Could you check a few things on this model? Use its own coordinates, in mm. Face numbers are marked on the shaded views. A direction names the side the tool comes from. Coordinates: 2 decimals unless noted, no trailing zeros. Order: outer loops, then holes, each group sorted by start corner. A loop starts at its lowest first (then second) coordinate and runs counter-clockwise, first axis right, second up. Notation, with made-up numbers: (-37.5, 64.25) - (-6.5, 64.25) arc R26 cw to (-6.5, 94.25) - close; hole circle Ø6 at (76.5, -26.5). An arc over 180 degrees is marked (long way). Answer as CSV lines item,"result". Start each with the question number.
1. For pin 1 (1.6 mm diameter, centred on x = 0, z = 0, fed in from +Y); pin 2 (2 mm diameter, centred on y = 6, z = -0.5, fed in from +X), each with a flat end and sliding along its axis, tell me the tip position at first contact or that it passes through.
2. Thinking about a two-plate mould opening in X: for the marked faces 3, 4 and 5, which applies, released by +X, released by -X, zero draft, split by the parting line, or undercut?
3. I want a section at A-A, the plane x = 0. List the corners of the cut face in (y, z) for me (3 decimals).
4. I want a section at B-B, the plane y = 1.5. List the corners of the cut face in (x, z) for me, and give its area (3 significant figures).
5. I need wall thicknesses on probe 1 along Y at (x, z) = (0, -1.25); probe 2 along Y at (x, z) = (0, 0.85); probe 3 along X at (y, z) = (7, -2.1). Which ranges of each line are inside material? Lowest first, please.
6. I want a section at C-C, the plane z = 0.65. List the corners of the cut face in (x, y) for me.
7. For the marked faces 1 and 2, which set-ups out of +Z, -Z, +X, -X, +Y, -Y let a thin tool reach every point of the face, with its end or its side?
8. I want a section at D-D, the plane y = 6. List the corners of the cut face in (x, z) for me (3 decimals).
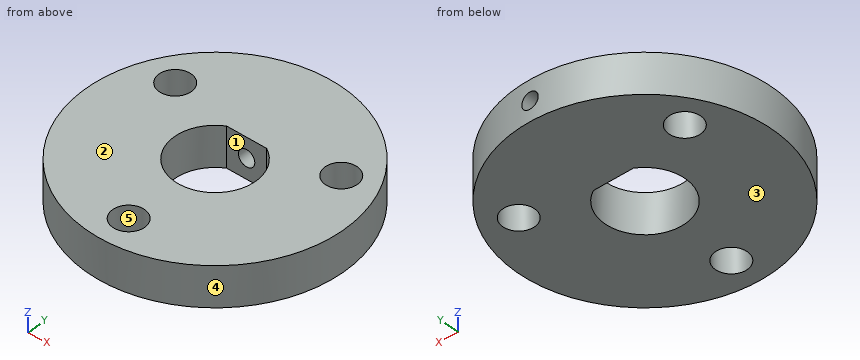
from build123d import *

# Parameters (mm, degrees)
SKETCH1_R            = 16
BOSS_EXTRUDE1_DEPTH  = 2.5
M4_CLEARANCE_HOLE2_D = 4
CIRPATTERN1_COUNT    = 3
SKETCH7_W            = 1.025
SKETCH7_H            = 11.612232914


with BuildPart() as part:
    # Sketch1 → Boss-Extrude1 (new body, symmetric)
    with BuildSketch(Plane.XY):
        Circle(SKETCH1_R)
        with BuildLine():
            Line((-2.5, 4.387767086), (2.5, 4.387767086))
            ThreePointArc((2.5, 4.387767086), (0, -5.05), (-2.5, 4.387767086))
        make_face(mode=Mode.SUBTRACT)
    extrude(amount=BOSS_EXTRUDE1_DEPTH, both=True)

    # M4 Clearance Hole2 (through all)
    with Locations(Plane.XY.offset(2.5)):
        with Locations((0, -12)):
            m4_clearance_hole2 = Hole(M4_CLEARANCE_HOLE2_D / 2)

    # CirPattern1: M4 Clearance Hole2 ×3 about axis
    cirpattern1_axis = Axis((0, 0, 0), (0, 0, 1))
    for i in range(1, CIRPATTERN1_COUNT):
        add(m4_clearance_hole2.rotate(cirpattern1_axis, i * 360 / CIRPATTERN1_COUNT), mode=Mode.SUBTRACT)

    # Sketch7 → M2.5x0.45 Tapped Hole1 (revolve, cut)
    with BuildSketch(Plane(origin=(0, 4.387767086, 0), x_dir=(0, 0, -1), z_dir=(1, 0, 0))):
        with Locations((0.5125, 5.806116457)):
            Rectangle(SKETCH7_W, SKETCH7_H)
    revolve(axis=Axis((0, -1.962232914, 0), (0, 1, 0)), mode=Mode.SUBTRACT)


solid = part.part
Solved:
1,pin 1,"stops at y = -4.99"
1,pin 2,"stops at x = 15.2"
2,face 3,"zero draft"
2,face 4,"split by the parting line"
2,face 5,"undercut"
3,outline,"(-16, -2.5) - (-14, -2.5) - (-14, 2.5) - (-16, 2.5) - close; (-10, -2.5) - (-5.05, -2.5) - (-5.05, 2.5) - (-10, 2.5) - close; (4.388, -2.5) - (16, -2.5) - (16, -1.025) - (4.388, -1.025) - close; (4.388, 1.025) - (16, 1.025) - (16, 2.5) - (4.388, 2.5) - close"
4,outline,"(-15.93, -2.5) - (-4.82, -2.5) - (-4.82, 2.5) - (-15.93, 2.5) - close; (4.82, -2.5) - (15.93, -2.5) - (15.93, 2.5) - (4.82, 2.5) - close"
4,area,"111 mm2"
5,probe 1,"y = -16 to -14, -10 to -5.05, 4.39 to 16"
5,probe 2,"y = -16 to -14, -10 to -5.05"
5,probe 3,"x = -14.39 to -12.12, -8.66 to 8.66, 12.12 to 14.39"
6,outline,"(-2.5, 4.39) - (-0.79, 4.39) - (-0.79, 15.98) arc R16 ccw (long way) to (0.79, 15.98) - (0.79, 4.39) - (2.5, 4.39) arc R5.05 cw (long way) to start; hole circle Ø4 at (-10.39, 6); hole circle Ø4 at (0, -12); hole circle Ø4 at (10.39, 6)"
7,face 1,"+Z, -Z"
7,face 2,"+Z, +X, -X, +Y, -Y"
8,outline,"(-14.832, -2.5) - (-12.392, -2.5) - (-12.392, 2.5) - (-14.832, 2.5) - close; (-8.392, -2.5) - (8.392, -2.5) - (8.392, 2.5) - (-8.392, 2.5) - close; (12.392, -2.5) - (14.832, -2.5) - (14.832, 2.5) - (12.392, 2.5) - close; hole circle Ø2.05 at (0, 0)"
